Here's how the part is built. I have some questions about the finished solid (model axes, mm). A direction names the side the tool comes from. Round coordinates to 2 decimals unless told otherwise and drop trailing zeros. Loops run counter-clockwise (first coordinate to the right, second up) from the corner with the lowest first, then second, coordinate; pieces in that order, holes last. Notation, with made-up numbers: M 22,55 L 39,55 A25 ccw 39,94 Z; hole C 58.5,72 d6. An arc over 180 degrees is marked long. Use a Markdown table: item, result.
Autodesk Inventor part; units mm, degrees
ref_plane "YZ Plane" through (0, 0, 0) normal (1, 0, 0) x (0, 1, 0)
ref_plane "XZ Plane" through (0, 0, 0) normal (0, 1, 0) x (-1, 0, 0)
ref_plane "XY Plane" through (0, 0, 0) normal (0, 0, 1) x (1, 0, 0)
sketch "Sketch1" plane through (0, 0, 0) normal (0, 1, 0) x (-1, 0, 0)
  line L0 (37.9, -17.5) -> (37.9, 17.5)
  line L1 (37.9, 17.5) -> (-37.9, 17.5)
  line L2 (-37.9, 17.5) -> (-37.9, -17.5)
  line L3 (37.9, -17.5) -> (14.9, -17.5)
  line L4 (14.9, -17.5) -> (14.9, -3.5)
  line L5 (14.9, -3.5) -> (-15, -3.5)
  line L6 (-15, -3.5) -> (-15, -17.5)
  line L7 (-37.9, -17.5) -> (-15, -17.5)
  line L8 (14.9, -17.5) -> (37.9, -17.5)
  circle A0 centre (-0.019, 9.5) radius 2.25
  circle A1 centre (-0.0381, 1.5) radius 2.25
  circle A2 centre (18.9586, -12.5) radius 2.25
  circle A3 centre (-19.0414, -12.5) radius 2.25
  circle A4 centre (-19.0414, 12.5) radius 2.25
  circle A5 centre (18.9586, 12.5) radius 2.25
  line L9 (18.9586, -12.5) -> (-19.0414, -12.5)
  line L10 (5.1, -12.5) -> (-13.9, -12.5)
  point P0 (0, 0)
  dimension "d0" = 75.8
  dimension "d1" = 35
  dimension "d2" = 23
  dimension "d3" = 14
  dimension "d4" = 29.9
  dimension "d7" = 4.5
  dimension "d8" = 4.5
  dimension "d11" = 4.5
  dimension "d12" = 4.5
  dimension "d20" = 38
  dimension "d21" = 0
  dimension "d23" = 38
extrude "Extrusion1" add sketch "Sketch1" along normal blind 18 contours L3 L4 L5 L6 L7 L2 L1 L0
chamfer "Chamfer1" distance 1 angle 45 8 edges at (-37.9, 18, 0) (0, 18, 17.5) (37.9, 18, 0) (-26.4, 18, -17.5) (26.45, 18, -17.5) (-14.9, 18, -10.5) (0.05, 18, -3.5) (15, 18, -10.5)
properties part number "GROUNDPLATE PART 1" material "Steel ASTM A36"
1. Imagine slicing it at C-C, the plane x = 0. Write out the boundary of the cut face in (y, z), then the cut area to 3 significant figures.
Answer sheet:
| item | result |
|---|---|
| outline | M 0,-3.5 L 17,-3.5 L 18,-2.5 L 18,-0.75 L 0,-0.75 Z; M 0,3.75 L 18,3.75 L 18,7.25 L 0,7.25 Z; M 0,11.75 L 18,11.75 L 18,16.5 L 17,17.5 L 0,17.5 Z |
| area | 215 mm2 |
2. For pin 1 Ø1.5 at (x, y) = (10, 15) entering from -Z, with a flat end and sliding along its axis, tell me the tip position at first contact or that it passes through.
Answer sheet:
| item | result |
|---|---|
| pin 1 | z = -3.5 |
3. I need wall thicknesses on probe 1 along X at (y, z) = (11, -7.5); probe 2 along Z at (x, y) = (20, 7); probe 3 along Z at (x, y) = (3, 9.5). Which ranges of each line are inside material? Lowest first, please. Write a range as from..to.
Answer sheet:
| item | result |
|---|---|
| probe 1 | -37.9..-14.9, 15..37.9 |
| probe 2 | -17.5..-14.54, -10.46..10.46, 14.54..17.5 |
| probe 3 | -3.5..17.5 |
4. Imagine slicing it at B-B, the plane y = 11.75. Write out the boundary of the cut face in (x, z), then the cut area to 3 significant figures.
Answer sheet:
| item | result |
|---|---|
| outline | M -37.9,-17.5 L -14.9,-17.5 L -14.9,-3.5 L 15,-3.5 L 15,-17.5 L 37.9,-17.5 L 37.9,17.5 L -37.9,17.5 Z; hole C -18.96,-12.5 d4.5; hole C -18.96,12.5 d4.5; hole C 0.02,9.5 d4.5; hole C 0.04,1.5 d4.5; hole C 19.04,-12.5 d4.5; hole C 19.04,12.5 d4.5 |
| area | 2,140 mm2 |
5. Imagine slicing it at D-D, the plane z = 12.5. Write out the boundary of the cut face in (x, y).
Answer sheet:
| item | result |
|---|---|
| outline | M -37.9,0 L -21.21,0 L -21.21,18 L -36.9,18 L -37.9,17 Z; M -16.71,0 L 16.79,0 L 16.79,18 L -16.71,18 Z; M 21.29,0 L 37.9,0 L 37.9,17 L 36.9,18 L 21.29,18 Z |
6. Imagine slicing it at A-A, the plane z = -12.5. Write out the boundary of the cut face in (x, y), then the cut area to 3 significant figures.
Answer sheet:
| item | result |
|---|---|
| outline | M -37.9,0 L -21.21,0 L -21.21,18 L -36.9,18 L -37.9,17 Z; M -16.71,0 L -14.9,0 L -14.9,17 L -15.9,18 L -16.71,18 Z; M 15,0 L 16.79,0 L 16.79,18 L 16,18 L 15,17 Z; M 21.29,0 L 37.9,0 L 37.9,17 L 36.9,18 L 21.29,18 Z |
| area | 662 mm2 |
7. Which directions (+Z, -Z, +X, -X, +Y, -Y) give clear straight access to the entire face, cutting with the end or side of a thin tool? Please do faces 1 (the face through (0.31, 8.87, 7.27)), 2 (the face through (0, 8, -3.5)).
Answer sheet:
| item | result |
|---|---|
| face 1 | +Y, -Y |
| face 2 | -Z, +Y, -Y |
